```python
from build123d import *

# Parameters (mm, degrees)
SKETCH_1_R               = 11
EXTRUDE_1_DEPTH          = 8
FILLET_1_R               = 100
FILLET_3_R               = 100
EXTRUDE_2_DEPTH          = 10
FILLET_2_R               = 10
CHAMFER_1_SIZE           = 5
SKETCH_4_R               = 13
CUT_EXTRUDE_1_DEPTH      = 0.7
SKETCH_5_R               = 2.75
CUT_EXTRUDE_2_DEPTH      = 514.540365546
SKETCH_6_R               = 6
CUT_EXTRUDE_3_DEPTH      = 4
CUT_EXTRUDE_4_DEPTH      = 514.758413114
CUT_EXTRUDE_4_DEPTH_BACK = 514.758413114
SKETCH_7_R               = 4.3


with BuildPart() as part:
    # 草图1 → 凸台-拉伸1 (new body)
    with BuildSketch(Plane.XY):
        Polygon((0, 280), (861.751390409, 0), (0, 0), (-100, 0), (-961.751390409, 0), (-100, 280), align=None)
        with Locations((200, 100)):
            Circle(SKETCH_1_R, mode=Mode.SUBTRACT)
        with Locations(Location((-300, 100, 0), (0, 0, 180))):
            Circle(SKETCH_1_R, mode=Mode.SUBTRACT)
    extrude(amount=EXTRUDE_1_DEPTH)

    # 圆角1
    fillet_1_edges = [part.edges().sort_by_distance(p)[0] for p in [
        (861.751390409, 0, 4),
    ]]
    fillet(fillet_1_edges, radius=FILLET_1_R)

    # 圆角3
    fillet_3_edges = [part.edges().sort_by_distance(p)[0] for p in [
        (-961.751390409, 0, 4),
    ]]
    fillet(fillet_3_edges, radius=FILLET_3_R)

    # 草图2 → 凸台-拉伸2 (add)
    with BuildSketch(Plane.XY):
        with BuildLine():
            Line((0, 280), (-100, 280))
            Line((-100, 280), (-361.277938379, 195.10565163))
            ThreePointArc((-361.277938379, 195.10565163), (-429.145073001, 84.356553496), (-330.376238942, 0))
            Line((-330.376238942, 0), (230.376238942, 0))
            ThreePointArc((230.376238942, 0), (329.145073001, 84.356553496), (261.277938379, 195.10565163))
            Line((261.277938379, 195.10565163), (0, 280))
        make_face()
        Polygon((10, 266.236180795), (122.241374643, 229.766747442), (10, 35.358983849), align=None, mode=Mode.SUBTRACT)
        with BuildLine():
            Line((230.376238942, 10), (30, 10))
            Line((30, 10), (151.410485182, 220.289128906))
            Line((151.410485182, 220.289128906), (258.187768435, 185.595086467))
            ThreePointArc((258.187768435, 185.595086467), (319.268189595, 85.920898146), (230.376238942, 10))
        make_face(mode=Mode.SUBTRACT)
        Polygon((-110, 266.236180795), (-110, 35.358983849), (-222.241374643, 229.766747442), align=None, mode=Mode.SUBTRACT)
        with BuildLine():
            Line((-358.187768435, 185.595086467), (-251.410485182, 220.289128906))
            Line((-251.410485182, 220.289128906), (-130, 10))
            Line((-130, 10), (-330.376238942, 10))
            ThreePointArc((-330.376238942, 10), (-419.268189595, 85.920898146), (-358.187768435, 185.595086467))
        make_face(mode=Mode.SUBTRACT)
    extrude(amount=-EXTRUDE_2_DEPTH)

    # 圆角2
    fillet_2_edges = [part.edges().sort_by_distance(p)[0] for p in [
        (-110, 35.358983849, -5),
        (-110, 266.236180795, -5),
        (-130, 10, -5),
        (10, 266.236180795, -5),
        (10, 35.358983849, -5),
        (151.410485182, 220.289128906, -5),
        (30, 10, -5),
        (-251.410485182, 220.289128906, -5),
        (122.241374643, 229.766747442, -5),
        (-222.241374643, 229.766747442, -5),
    ]]
    fillet(fillet_2_edges, radius=FILLET_2_R)

    # 倒角1
    chamfer_1_edges = [part.edges().sort_by_distance(p)[0] for p in [
        (-230.63896919, 237.552825815, 8),
        (130.63896919, 237.552825815, 8),
        (329.145073001, 84.356553496, 8),
        (-50, 0, 8),
        (-429.145073001, 84.356553496, 8),
        (-230.63896919, 237.552825815, -10),
        (130.63896919, 237.552825815, -10),
        (329.145073001, 84.356553496, -10),
        (-50, 0, -10),
        (-429.145073001, 84.356553496, -10),
    ]]
    chamfer(chamfer_1_edges, length=CHAMFER_1_SIZE)

    # 草图4 → 切除-拉伸1 (cut)
    with BuildSketch(Plane(origin=(0, 0, 0), x_dir=(-1, 0, 0), z_dir=(0, 0, -1))):
        with Locations((-200, 100)):
            Circle(SKETCH_4_R)
        with Locations((300, 100)):
            Circle(SKETCH_4_R)
    extrude(amount=-CUT_EXTRUDE_1_DEPTH, mode=Mode.SUBTRACT)

    # 草图5 → 切除-拉伸2 (cut, through all)
    with BuildSketch(Plane(origin=(0, 0, 0), x_dir=(-1, 0, 0), z_dir=(0, 0, -1))):
        with Locations((-200, 130)):
            Circle(SKETCH_5_R)
        with Locations((-200, 70)):
            Circle(SKETCH_5_R)
        with Locations((300, 130)):
            Circle(SKETCH_5_R)
        with Locations((300, 70)):
            Circle(SKETCH_5_R)
    extrude(amount=-CUT_EXTRUDE_2_DEPTH, mode=Mode.SUBTRACT)

    # 草图6 → 切除-拉伸3 (cut)
    with BuildSketch(Plane.XY.offset(8)):
        with Locations((200, 130)):
            Circle(SKETCH_6_R)
        with Locations((200, 70)):
            Circle(SKETCH_6_R)
    extrude(amount=-CUT_EXTRUDE_3_DEPTH, mode=Mode.SUBTRACT)

    # 草图7 → 切除-拉伸4 (cut, two sides: drawn at the far end of the back side and taken through both)
    with BuildSketch(Plane.XY.offset(8).offset(-CUT_EXTRUDE_4_DEPTH_BACK)):
        with Locations((64, 217)):
            Circle(SKETCH_7_R)
        with Locations((24, 217)):
            Circle(SKETCH_7_R)
        with Locations((64, 177)):
            Circle(SKETCH_7_R)
        with Locations((24, 177)):
            Circle(SKETCH_7_R)
        with Locations((64, 89)):
            Circle(SKETCH_7_R)
        with Locations((24, 89)):
            Circle(SKETCH_7_R)
        with Locations((64, 49)):
            Circle(SKETCH_7_R)
        with Locations((24, 49)):
            Circle(SKETCH_7_R)
        with Locations(Location((-124, 49, 0), (0, 0, 180))):
            Circle(SKETCH_7_R)
        with Locations(Location((-164, 49, 0), (0, 0, 180))):
            Circle(SKETCH_7_R)
        with Locations(Location((-124, 89, 0), (0, 0, 180))):
            Circle(SKETCH_7_R)
        with Locations(Location((-164, 89, 0), (0, 0, 180))):
            Circle(SKETCH_7_R)
        with Locations(Location((-124, 177, 0), (0, 0, 180))):
            Circle(SKETCH_7_R)
        with Locations(Location((-164, 177, 0), (0, 0, 180))):
            Circle(SKETCH_7_R)
        with Locations(Location((-124, 217, 0), (0, 0, 180))):
            Circle(SKETCH_7_R)
        with Locations(Location((-164, 217, 0), (0, 0, 180))):
            Circle(SKETCH_7_R)
    extrude(amount=CUT_EXTRUDE_4_DEPTH + CUT_EXTRUDE_4_DEPTH_BACK, mode=Mode.SUBTRACT)


solid = part.part
```
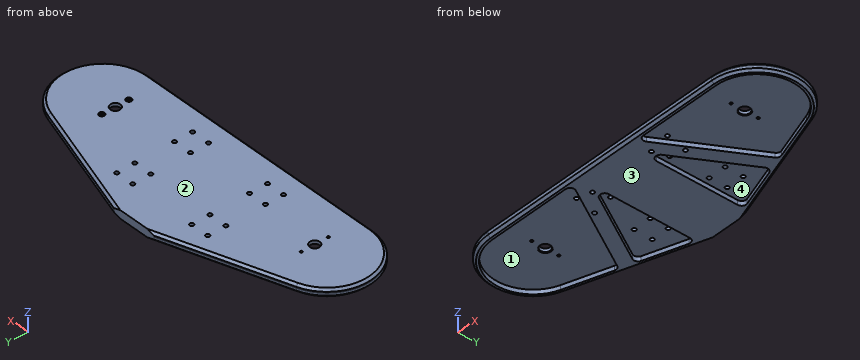
Geometry: final body of the model. Coordinates: model frame, mm. Face numbers are marked on the shaded views. A direction names the side the tool comes from. Round coordinates to 2 decimals unless told otherwise and drop trailing zeros. Write item = value, one per line. Start each with the question number.
Q1. Pin query (flat end, axial travel): pin 1 (5 mm diameter, centred on x = -124, y = 89, fed in from -Z); pin 2 (3 mm diameter, centred on x = -241, y = 191.5, fed in from -Z); pin 3 (4 mm diameter, centred on y = 118, z = -7, fed in from +X); pin 4 (5 mm diameter, centred on y = 144, z = 1.5, fed in from -X). Return the tip coordinate at first contact, or that it passes through.
Q2. Ray query, line 1 (X direction, y = 137, z = -7); line 2 (X direction, y = 63.5, z = -7.5); line 3 (Y direction, x = -300, z = 0.45). Return the intervals inside material, ascending. Write a range as from..to.
Q3. Pull-direction query (X, two-part tool) for the marked faces 3 and 4; classes: +X half, -X half, draft (parallel to the pull), parting line (faces both ways), or undercut.
Q4. Access query for the marked faces 1 and 2. Directions: +Z, -Z, +X, -X, +Y, -Y. A direction counts if a zero-diameter tool reaches every point of the face in a straight line with its end or side. Return the directions, or none.
Outcome:
q1.pin_1 = through
q1.pin_2 = 0
q1.pin_3 = 328.77
q1.pin_4 = -421.36
q2.line_1 = -421.12..-412.42, -203.32..-168.68, -110..10, 68.68..103.32, 312.42..321.12
q2.line_2 = -420.79..-412.64, -160.89..-123.97, -116.03..16.03, 23.97..60.89, 312.64..320.79
q2.line_3 = 0..67.25, 72.75..87, 113..127.25, 132.75..215.02
q3.face_3 = draft
q3.face_4 = undercut
q4.face_1 = -Z
q4.face_2 = +Z, +X, -X, +Y, -Y
